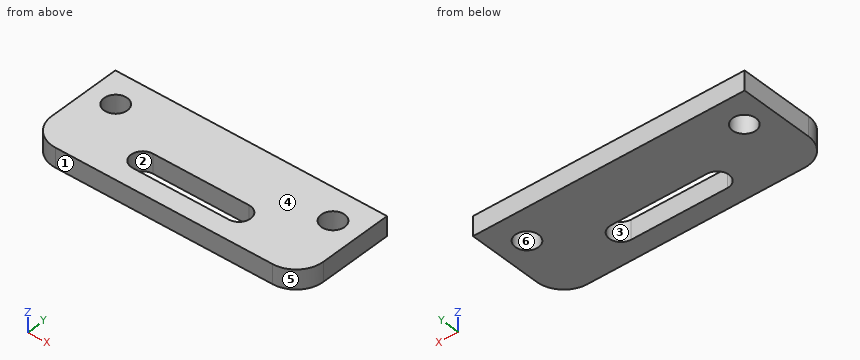
from build123d import *

# Parameters (mm, degrees)
SKETCH1_R           = 1
SKETCH1_R_2         = 1.5
SKETCH1_R_3         = 2
SKETCH1_W           = 23
SKETCH1_H           = 12
BOSS_EXTRUDE1_DEPTH = 2.5
FILLET1_R           = 3.5
SKETCH2_W           = 57.93350489
SKETCH2_H           = 33.625772429
CUT_EXTRUDE1_DEPTH  = 10


with BuildPart() as part:
    # Sketch1 → Boss-Extrude1 (new body)
    with BuildSketch(Plane.XY):
        with BuildLine():
            Line((-17.5, 9), (-17.5, -19))
            Line((-17.5, -19), (17.5, -19))
            Line((17.5, -19), (17.5, 9))
            ThreePointArc((17.5, 9), (0, 26), (-17.5, 9))
        make_face()
        with Locations((-14, 0)):
            Circle(SKETCH1_R, mode=Mode.SUBTRACT)
        with Locations((-14, -10)):
            Circle(SKETCH1_R_2, mode=Mode.SUBTRACT)
        with Locations((-8.5, 16)):
            Circle(SKETCH1_R_3, mode=Mode.SUBTRACT)
        with Locations((14, -10)):
            Circle(SKETCH1_R_2, mode=Mode.SUBTRACT)
        with Locations((14, 0)):
            Circle(SKETCH1_R, mode=Mode.SUBTRACT)
        with Locations((8.5, 16)):
            Circle(SKETCH1_R_3, mode=Mode.SUBTRACT)
        Rectangle(SKETCH1_W, SKETCH1_H, mode=Mode.SUBTRACT)
        with BuildLine():
            Line((-6.2, -13.5), (6.2, -13.5))
            ThreePointArc((6.2, -13.5), (7.7, -15), (6.2, -16.5))
            Line((6.2, -16.5), (-6.2, -16.5))
            ThreePointArc((-6.2, -16.5), (-7.7, -15), (-6.2, -13.5))
        make_face(mode=Mode.SUBTRACT)
    extrude(amount=BOSS_EXTRUDE1_DEPTH)

    # Fillet1
    fillet1_edges = [part.edges().sort_by_distance(p)[0] for p in [
        (17.5, -19, 1.25),
        (-17.5, -19, 1.25),
    ]]
    fillet(fillet1_edges, radius=FILLET1_R)

    # Sketch2 → Cut-Extrude1 (cut)
    with BuildSketch(Plane.XY.offset(2.5)):
        with Locations((-1.18759747, 10.812886215)):
            Rectangle(SKETCH2_W, SKETCH2_H)
    extrude(amount=-CUT_EXTRUDE1_DEPTH, mode=Mode.SUBTRACT)


solid = part.part
Could you check a few things on this model? Use its own coordinates, in mm. Face numbers are marked on the shaded views. A direction names the side the tool comes from. Round coordinates to 2 decimals unless told otherwise and drop trailing zeros. Order: outer loops, then holes, each group sorted by start corner. A loop starts at its lowest first (then second) coordinate and runs counter-clockwise, first axis right, second up.
(1) Please list where these lines run through material, in increasing order: line 1 along Y through (x, z) = (6, 0.4); line 2 along X through (y, z) = (-9, 1.5); line 3 along X through (y, z) = (-11.25, 1).
Response values:
line 1: y = -19 to -16.5, -13.5 to -6
line 2: x = -17.5 to -15.12, -12.88 to 12.88, 15.12 to 17.5
line 3: x = -17.5 to -14.83, -13.17 to 13.17, 14.83 to 17.5
(2) Which directions (+Z, -Z, +X, -X, +Y, -Y) give clear straight access to the entire face, cutting with the end or side of a thin tool? Please do the marked faces 1 and 2.
Response values:
face 1: +Z, -Z, +X, -X, -Y
face 2: +Z, -Z
(3) Imagine slicing it at C-C (z = 0.65). Write out the boundary of the cut face in (x, y).
Response values:
outline: (-17.5, -15.5) arc R3.5 ccw to (-14, -19) - (14, -19) arc R3.5 ccw to (17.5, -15.5) - (17.5, -6) - (-17.5, -6) - close; hole circle Ø3 at (-14, -10); hole (-6.2, -16.5) - (6.2, -16.5) arc R1.5 ccw to (6.2, -13.5) - (-6.2, -13.5) arc R1.5 ccw to start; hole circle Ø3 at (14, -10)
(4) Imagine slicing it at A-A (y = -15). Write out the boundary of the cut face in (x, z), plus the area to 3 significant figures.
Response values:
outline: (-17.5, 0) - (-7.7, 0) - (-7.7, 2.5) - (-17.5, 2.5) - close; (7.7, 0) - (17.5, 0) - (17.5, 2.5) - (7.7, 2.5) - close
area: 49.0 mm2
(5) I'm going to push a flat-ended pin straight in: pin 1 (5 mm diameter, centred on x = 14, y = -10, fed in from +Z). Where does the tip first touch, or does it pass through?
Response values:
pin 1: stops at z = 2.5
(6) Imagine slicing it at B-B (x = 1). Write out the boundary of the cut face in (y, z), plus the area to 3 significant figures.
Response values:
outline: (-19, 0) - (-16.5, 0) - (-16.5, 2.5) - (-19, 2.5) - close; (-13.5, 0) - (-6, 0) - (-6, 2.5) - (-13.5, 2.5) - close
area: 25.0 mm2
(7) If we mould it in two halves opening along X, with no side actions, what happens to the marked faces 3, 4, 5 and 6? For each: released by +X, released by -X, zero draft, split by the parting line, or undercut.
Response values:
face 3: undercut
face 4: zero draft
face 5: released by +X
face 6: undercut
(8) Imagine slicing it at D-D (y = -10). Write out the boundary of the cut face in (x, z).
Response values:
outline: (-17.5, 0) - (-15.5, 0) - (-15.5, 2.5) - (-17.5, 2.5) - close; (-12.5, 0) - (12.5, 0) - (12.5, 2.5) - (-12.5, 2.5) - close; (15.5, 0) - (17.5, 0) - (17.5, 2.5) - (15.5, 2.5) - close
